Model file for the job. Use its own axes, mm. A direction names the side the tool comes from. Give positions to 0.01 mm unless a question says otherwise; leave off trailing zeros. Order: outer loops, then holes, each group sorted by start corner. A loop starts at its lowest first (then second) coordinate and runs counter-clockwise, first axis right, second up. Notation, with made-up numbers: (85, 8) -> (118, 8) arc R16 cw to (118, 15) -> close; hole circle Ø7 at (-23.5, 74.25). An arc over 180 degrees is marked (long way). Answer in a Markdown table with one row per item. Add a question column.
from build123d import *

# Parameters (mm, degrees)
F4_SIZE  = 2
F5_R     = 4.99999
F6_DEPTH = 5


# Not quite as in the source:
# - a fillet or chamfer is up to 0.001 mm smaller than in the source, because OpenCascade refuses the exact size


with BuildPart() as f1:
    # F0 (on Right) → F1 (revolve)
    with BuildSketch(Plane.YZ):
        Polygon((8.0283725262, 25), (0, 25), (-71.9716274738, 25), (-71.9716274738, 20), (-131.9716274738, 20), (-131.9716274738, 0), (48.0283725262, 0), (48.0283725262, 20), (8.0283725262, 20), align=None)
    revolve(axis=Axis((0, -30.3001217544, 0), (0, 1, 0)))

    # F4
    f4_edges = [f1.edges().sort_by_distance(p)[0] for p in [
        (0, -131.971627, -20),
        (0, 48.028373, -20),
    ]]
    chamfer(f4_edges, length=F4_SIZE)

    # F5 (radius 5 in the source; OpenCascade refuses exactly that, so slightly less here)
    f5_edges = [f1.edges().sort_by_distance(p)[0] for p in [
        (0, -71.971627, -20),
        (0, 8.028373, -20),
    ]]
    fillet(f5_edges, radius=F5_R)

    # F3 (on offset) → F6 (cut)
    with BuildSketch(Plane.YZ.offset(25)):
        with BuildLine():
            Line((-16.4436194198, 6), (-46.4436194198, 6))
            ThreePointArc((-46.4436194198, 6), (-52.4436194198, 0), (-46.4436194198, -6))
            Line((-46.4436194198, -6), (-16.4436194198, -6))
            ThreePointArc((-16.4436194198, -6), (-10.4436194198, 0), (-16.4436194198, 6))
        make_face()
    extrude(amount=-F6_DEPTH, mode=Mode.SUBTRACT)


solid = f1.part
Item 1: Two-plate mould, pull along Y, no slides. Class faces 4 (the flat face through (0, -131.972, 0)), 5 (the flat face through (20, -32, 0)), 6 (the cylindrical face through (-19.524, -103.843, -4.336)): pulls with the +Y half, pulls with the -Y half, needs draft (parallel to the pull), parting line crosses it, or undercut.
Item 2: Saw through at C-C on y = -88. List the corners of the cut face in (x, z), plus the area to 3 significant figures.
Item 3: Wall check: line 1 (Z direction, x = 23, y = -20); line 2 (X direction, y = -119, z = 0); line 3 (Y direction, x = 23.5, z = -3.5). Give the ranges that are in metal, low to high.
Item 4: Pin check, flat tips, straight feed: pin 1 Ø1 at (y, z) = (-69.5, 15) entering from +X; pin 2 Ø1.5 at (y, z) = (-69, -19) entering from -X; pin 3 Ø3.5 at (x, y) = (22.5, -25) entering from -Z. Stop position of each tip, or through.
Item 5: Saw through at D-D on y = -12.5. List the corners of the cut face in (x, z), plus the area to 3 significant figures.
Item 6: Which spindle directions (+Z, -Z, +X, -X, +Y, -Y) get a long thin tool onto all of the face, cutting with end or side? Do faces 1 (the flat face through (0, 48.028, 0)), 2 (the cylindrical face through (-19.524, 29.297, -4.336)), 3 (the cylindrical face through (22.536, -10.445, -0.132)). Say none if no direction does.
Evaluation:
| question | item | result |
|---|---|---|
| 1 | face 4 | pulls with the -Y half |
| 1 | face 5 | undercut |
| 1 | face 6 | needs draft |
| 2 | outline | circle Ø40 at (0, 0) |
| 2 | area | 1,260 mm2 |
| 3 | line 1 | z = -9.8 to -6, 6 to 9.8 |
| 3 | line 2 | x = -20 to 20 |
| 3 | line 3 | y = -72.13 to -51.32, -11.57 to 8.18 |
| 4 | pin 1 | stops at x = 20.37 |
| 4 | pin 2 | stops at x = -17.09 |
| 4 | pin 3 | stops at z = -13.94 |
| 5 | outline | (20, -4.52) -> (20, 4.52) -> (24.59, 4.52) arc R25 ccw (long way) to (24.59, -4.52) -> close |
| 5 | area | 1,920 mm2 |
| 6 | face 1 | +Z, -Z, +X, -X, +Y |
| 6 | face 2 | +Y |
| 6 | face 3 | +X |
